For this review, take the finished solid that the model builds, in its own axes (mm). Face numbers are marked on the shaded views. Coordinates: 2 decimals unless noted, no trailing zeros. Order: outer loops, then holes, each group sorted by start corner. A loop starts at its lowest first (then second) coordinate and runs counter-clockwise, first axis right, second up. Notation, with made-up numbers: (-28, 70.25) -> (2, 70.25) arc R9 ccw to (2, 76.25) -> close; hole circle Ø10 at (42.25, 34). An arc over 180 degrees is marked (long way). Write item = value, one per line. Start each with the question number.
1) Wall thickness on probe 1 along Y at (x, z) = (0, 8.75); probe 2 along X at (y, z) = (-1.75, 1.25); probe 3 along Y at (x, z) = (6.5, 4.25): over which ranges is each line inside the solid? List them lowest first. Write a range as [from, to].
2) Insertion check: pin 1 Ø1 at (y, z) = (9, 6.5) entering from +X; pin 2 Ø2 at (y, z) = (1.5, 2.5) entering from +X; pin 3 Ø5 at (x, y) = (0, 0) entering from -Z. Each pin has a flat end and moves straight along its axis. Give the tip position at first contact, or say it passes through.
3) Draft analysis for pull direction Y (two halves, no side actions). For the marked faces 1, 2 and 3, state which applies: +Y half, -Y half, draft (parallel to the pull), parting line (faces both ways), or undercut.
4) Consider section A-A on x = 0. Give the boundary of the cut face in (y, z).
5) Consider section C-C on z = 10. Give the boundary of the cut face in (x, y).
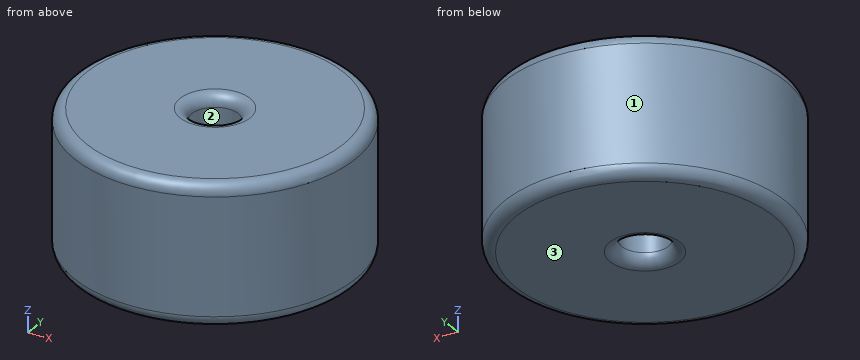
from build123d import *

# Parameters (mm, degrees)
SKETCH_1_R          = 12
EXTRUDE_1_DEPTH     = 12
FILLET_1_R          = 1
SKETCH_2_R          = 2
CUT_EXTRUDE_1_DEPTH = 12
FILLET_2_R          = 1


with BuildPart() as part:
    # 草图1 → 凸台-拉伸1 (new body)
    with BuildSketch(Plane.XY):
        Circle(SKETCH_1_R)
    extrude(amount=EXTRUDE_1_DEPTH)

    # 圆角1
    fillet_1_edges = [part.edges().sort_by_distance(p)[0] for p in [
        (-12, 0, 0),
        (-12, 0, 12),
    ]]
    fillet(fillet_1_edges, radius=FILLET_1_R)

    # 草图2 → 切除-拉伸1 (cut)
    with BuildSketch(Plane(origin=(0, 0, 0), x_dir=(-1, 0, 0), z_dir=(0, 0, -1))):
        Circle(SKETCH_2_R)
    extrude(amount=-CUT_EXTRUDE_1_DEPTH, mode=Mode.SUBTRACT)

    # 圆角2
    fillet_2_edges = [part.edges().sort_by_distance(p)[0] for p in [
        (2, 0, 12),
        (2, 0, 0),
    ]]
    fillet(fillet_2_edges, radius=FILLET_2_R)


solid = part.part
Answer sheet:
q1.probe_1 = [-12, -2], [2, 12]
q1.probe_2 = [-11.87, -0.97], [0.97, 11.87]
q1.probe_3 = [-10.09, 10.09]
q2.pin_1 = 8.47
q2.pin_2 = 11.99
q2.pin_3 = 0.13
q3.face_1 = parting line
q3.face_2 = undercut
q3.face_3 = draft
q4.outline = (-12, 1) arc R1 ccw to (-11, 0) -> (-3, 0) arc R1 ccw to (-2, 1) -> (-2, 11) arc R1 ccw to (-3, 12) -> (-11, 12) arc R1 ccw to (-12, 11) -> close; (2, 1) arc R1 ccw to (3, 0) -> (11, 0) arc R1 ccw to (12, 1) -> (12, 11) arc R1 ccw to (11, 12) -> (3, 12) arc R1 ccw to (2, 11) -> close
q5.outline = circle Ø24 at (0, 0); hole circle Ø4 at (0, 0)
